Build history of the part. All positions in model axes, mm. Round coordinates to 2 decimals unless told otherwise and drop trailing zeros. Loops run counter-clockwise (first coordinate to the right, second up) from the corner with the lowest first, then second, coordinate; pieces in that order, holes last. Notation, with made-up numbers: (29, 62) - (86, 62) arc R19 ccw to (86, 71) - close; hole circle Ø1 at (33.5, 64.5). An arc over 180 degrees is marked (long way). Put each result on its own line as item: value. Start each with the question number.
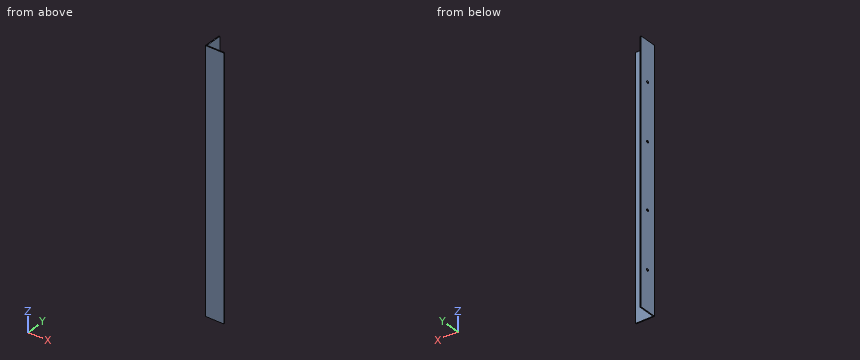
Autodesk Inventor part; units mm, degrees
ref_plane "YZ Plane" through (0, 0, 0) normal (1, 0, 0) x (0, 1, 0)
ref_plane "XZ Plane" through (0, 0, 0) normal (0, 1, 0) x (-1, 0, 0)
ref_plane "XY Plane" through (0, 0, 0) normal (0, 0, 1) x (1, 0, 0)
sketch "Sketch1" plane through (0, 0, 0) normal (0, 1, 0) x (-1, 0, 0)
  line L0 (0, 0) -> (0, -406.4)
  line L1 (0, -406.4) -> (27.94, -406.4)
  line L2 (27.94, -406.4) -> (27.94, 0)
  line L3 (27.94, 0) -> (0, 0)
  dimension "d0" = 406.4
  dimension "d1" = 27.94
extrude "Extrusion1" add sketch "Sketch1" along normal blind 1.524
sketch "Sketch2" plane through (0, 0, 0) normal (0, -1, 0) x (1, 0, 0)
  line L0 (-27.94, 0) -> (0, 0)
  line L1 (-27.94, 0) -> (-29.464, 0)
  line L2 (-29.464, 0) -> (-29.464, -406.4)
  line L3 (0, -406.4) -> (-27.94, -406.4)
  line L4 (-29.464, -406.4) -> (-27.94, -406.4)
  line L5 (-27.94, -406.4) -> (-27.94, 0)
  line L6 (-27.94, -406.4) -> (-27.94, 0)
  dimension "d4" = 1.524
extrude "Extrusion2" add sketch "Sketch2" against normal blind 27.94
sketch "Sketch3" plane through (-29.464, 0, -406.4) normal (-1, 0, 0) x (0, 0, 1)
  line L0 (406.4, 1.524) -> (0, 1.524)
  line L1 (203.2, 1.524) -> (166.37, 1.524)
  line L2 (203.2, 1.524) -> (240.03, 1.524)
  point P0 (406.4, 0)
  dimension "d7" = 36.83
  dimension "d8" = 36.83
sketch "Sketch4" plane through (-29.464, 0, -406.4) normal (-1, 0, 0) x (0, 0, 1)
  line L0 (0, 1.524) -> (0, 27.94)
  line L1 (0, 14.732) -> (406.4, 14.732)
  line L2 (406.4, 1.524) -> (406.4, 27.94)
  point P0 (406.4, 0)
sketch "Sketch6" plane through (-29.464, 0, -406.4) normal (-1, 0, 0) x (0, 0, 1)
  circle A0 centre (344.1078, 14.732) radius 1.905
  circle A1 centre (254.5728, 14.732) radius 1.905
  circle A2 centre (151.7515, 14.732) radius 1.905
  circle A3 centre (62.2165, 14.732) radius 1.905
  point P0 (406.4, 0)
extrude "Extrusion4" cut sketch "Sketch6" against normal blind 17.4625
properties part number "Flywheel Headpiece" material "Steel, Alloy"
1) Slice it at B-B, the plane x = -20.5. Write the cut outline in (y, z), and give its area (3 significant figures).
2) Slice it at C-C, the plane y = 22.75. Write the cut outline in (x, z).
3) Slice it at A-A, the plane z = -182.5. Write the cut outline in (x, y), and give its area (3 significant figures).
4) Drill centre lines: line 1 (Y direction, x = -23.5, z = -102); line 2 (X direction, y = 18.75, z = -302). Where is each one in solid material? Low to high. Write a range as [from, to].
5) Drop flat-ended pins along their axis: pin 1 Ø4 at (x, z) = (-20.5, -240) entering from +Y; pin 2 Ø8 at (y, z) = (14, -125.5) entering from +X. Give the stop position or say it passes through.
Taken from the geometry:
1. outline: (0, -406.4) - (1.52, -406.4) - (1.52, 0) - (0, 0) - close
1. area: 619 mm2
2. outline: (-29.46, -406.4) - (-27.94, -406.4) - (-27.94, 0) - (-29.46, 0) - close
3. outline: (-29.46, 0) - (0, 0) - (0, 1.52) - (-27.94, 1.52) - (-27.94, 27.94) - (-29.46, 27.94) - close
3. area: 85.2 mm2
4. line 1: y = [0, 1.52]
4. line 2: x = [-29.46, -27.94]
5. pin 1: stops at y = 1.52
5. pin 2: stops at x = -27.94
